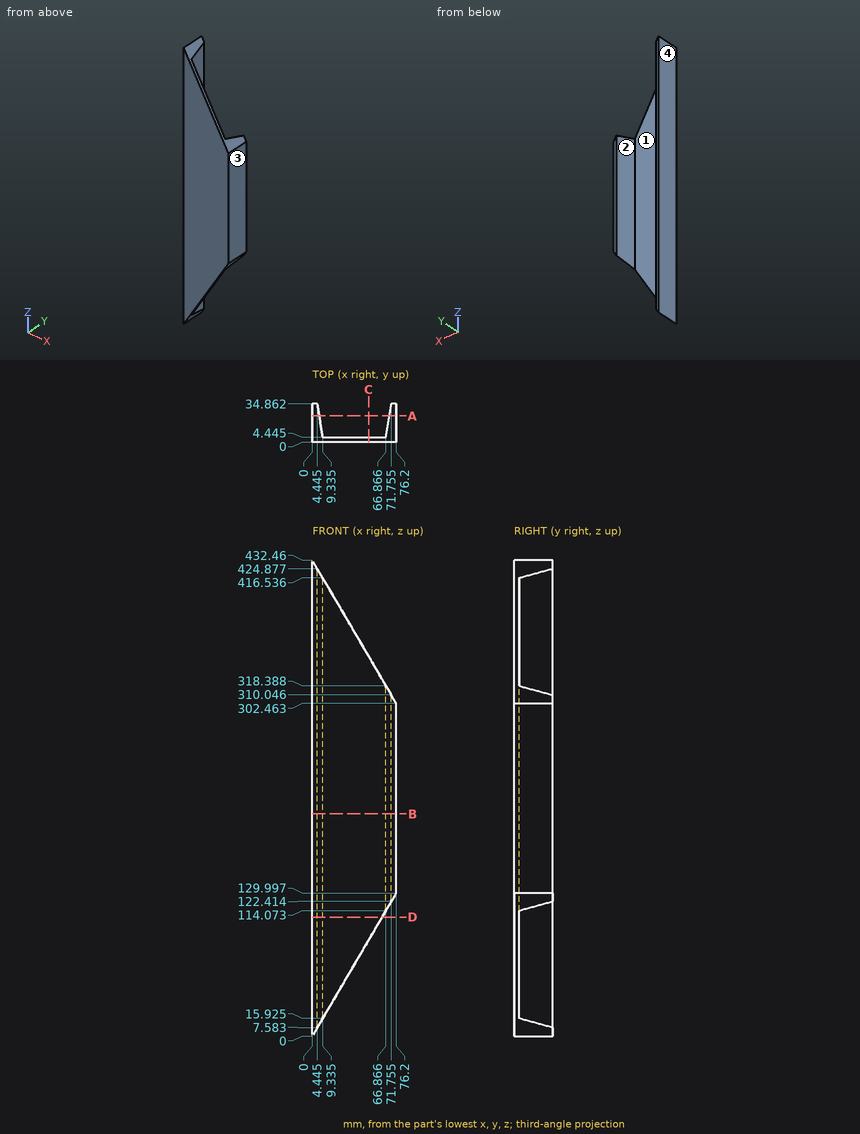
Geometry check sheet. Reference: drawing and pictorial views, mm from the part's lowest x, y, z. Round coordinates to 2 decimals unless told otherwise and drop trailing zeros. Loops run counter-clockwise (first coordinate to the right, second up) from the corner with the lowest first, then second, coordinate; pieces in that order, holes last.
1. Sectioned sample at C-C on x = 51. Record the boundary of the cut face in (y, z) (1 decimal).
2. Mould release check, pull along X, two halves, no side actions. Record for the marked faces 1, 2, 3 and 4: released by +X, released by -X, zero draft, split by the parting line, or undercut.
3. Sectioned sample at D-D on z = 108. Record the boundary of the cut face in (x, y) (1 decimal), and give its area (3 significant figures).
4. Gauge pin test, flat ends, axial feed: pin 1 Ø4 at (y, z) = (31.5, 45) entering from +X; pin 2 Ø5 at (x, z) = (44, 83.5) entering from +Y (1 decimal); pin 3 Ø4 at (x, y) = (56, 4) entering from +Z (1 decimal). Record the tip position at first contact, or that the pin passes through.
5. Sectioned sample at B-B on z = 202. Record the boundary of the cut face in (x, y) (1 decimal), and give its area (3 significant figures).
6. Scan lines: probe 1 along Y at (x, z) = (14, 225) (1 decimal); probe 2 along X at (y, z) = (28, 123.5); probe 3 along X at (y, z) = (31.5, 217.5) (1 decimal). Record each from-to range of solid material in increasing order.
7. Sectioned sample at A-A on y = 24. Record the boundary of the cut face in (x, z) (1 decimal).
Recorded:
1. outline: (0, 87) - (4.4, 87) - (4.4, 345.5) - (0, 345.5) - close
2. face 1: undercut
2. face 2: undercut
2. face 3: released by +X
2. face 4: released by -X
3. outline: (0, 0) - (63.3, 0) - (63.3, 4.4) - (9.3, 4.4) - (4.4, 34.9) - (0, 34.9) - close
3. area: 491 mm2
4. pin 1: stops at x = 5.31
4. pin 2: stops at y = 4.4
4. pin 3: stops at z = 340.3
5. outline: (0, 0) - (76.2, 0) - (76.2, 34.9) - (71.8, 34.9) - (66.9, 4.4) - (9.3, 4.4) - (4.4, 34.9) - (0, 34.9) - close
5. area: 758 mm2
6. probe 1: y = 0 to 4.4
6. probe 2: x = 0 to 5.55, 70.65 to 72.39
6. probe 3: x = 0 to 5, 71.2 to 76.2
7. outline: (0, 0) - (6.2, 10.6) - (6.2, 421.9) - (0, 432.5) - close; (70, 119.4) - (76.2, 130) - (76.2, 302.5) - (70, 313) - close
